Autodesk Inventor part; units mm, degrees
ref_plane "YZ Plane" through (0, 0, 0) normal (1, 0, 0) x (0, 1, 0)
ref_plane "XZ Plane" through (0, 0, 0) normal (0, 1, 0) x (-1, 0, 0)
ref_plane "XY Plane" through (0, 0, 0) normal (0, 0, 1) x (1, 0, 0)
sketch "Эскиз1" plane through (0, 0, 0) normal (0, 1, 0) x (-1, 0, 0)
  line L0 (0, 0) -> (12, 0)
  line L1 (12, 0) -> (12, -28)
  line L2 (12, -28) -> (0, -28)
  line L3 (0, -28) -> (0, 0)
  circle A0 centre (6, -12) radius 0.65
  circle A1 centre (6, -17) radius 2.5
  circle A2 centre (6, -22) radius 0.65
  line L4 (6, -12) -> (6, -17) construction
  line L5 (6, -17) -> (6, -22) construction
  line L6 (6, -6) -> (6, 0) construction
  line L7 (6, -12) -> (12, -12) construction
  circle A3 centre (6, -12) radius 1.15
  circle A4 centre (6, -22) radius 1.15
  line L8 (6, -22) -> (6, -28) construction
  line L9 (6, -12) -> (6, -6) construction
  point P0 (12, -14)
  dimension "d0" = 5
  dimension "d1" = 6
  dimension "d2" = 5
  dimension "d7" = 0.5
  dimension "d8" = 1.3
  dimension "d20" = 6
extrude "Выдавливание1" add sketch "Эскиз1" against normal blind 9 contours L0 L1 L2 L3 | A0 | A1 | A2 | A3 | A4
shell "Оболочка1" thickness 0.7 removed faces 1 at (-4, -9, -9.3333)
extrude "Выдавливание2" cut sketch "Эскиз1" against normal through all contours A0 | A1 | A2
sketch "Эскиз2" plane through (0, -9, 0) normal (0, -1, 0) x (1, 0, 0)
  line L0 (0, -28) -> (-12, -28) construction
  line L1 (-6, -28) -> (-6, 0) construction
  line L2 (-12, 0) -> (0, 0) construction
  line L3 (-12, -28) -> (-12, 0) construction
  line L4 (-12, -14) -> (0, -14) construction
  line L5 (0, 0) -> (0, -28) construction
  circle A0 centre (-1.1, -26.9) radius 0.9
  circle A1 centre (-1.1, -26.9) radius 0.5
  circle A2 centre (-10.9, -26.9) radius 0.9
  circle A3 centre (-10.9, -26.9) radius 0.5
  circle A4 centre (-1.1, -1.1) radius 0.9
  circle A5 centre (-1.1, -1.1) radius 0.5
  circle A6 centre (-10.9, -1.1) radius 0.5
  circle A7 centre (-10.9, -1.1) radius 0.9
  dimension "d11" = 1.1
  dimension "d12" = 1.1
  dimension "d13" = 1
  dimension "d14" = 0.4
extrude "Выдавливание3" cut sketch "Эскиз2" against normal through all contours A0 | A1 | A2 | A3 | A4 | A5 | A6 | A7
extrude "Выдавливание4" add sketch "Эскиз2" along normal blind 8.8 from surface at -9
fillet "Сопряжение1" radius 1 4 edges at (-12, -4.5, -28) (0, -4.5, -28) (0, -4.5, 0) (-12, -4.5, 0)
equation "\"d11\" = d12"
properties part number "Голова сервы"
Can you work these out from the model? Positions are in its coordinate system, mm. A direction names the side the tool comes from. Coordinates: 2 decimals unless noted, no trailing zeros. Loops run counter-clockwise (first coordinate to the right, second up) from the corner with the lowest first, then second, coordinate; pieces in that order, holes last.
1) Which directions (+Z, -Z, +X, -X, +Y, -Y) give clear straight access to the entire face, cutting with the end or side of a thin tool? Please do faces 1 (the flat face through (-6, -0.7, -14)), 2 (the cylindrical face through (-0.285, -4.563, -0.301)).
2) Imagine slicing it at D-D on x = -4.75. List the corners of the cut face in (y, z) for me, plus the area to 3 significant figures.
3) Thinking about a two-plate mould opening in Z: for faces 3 (the flat face through (-6, -4, -28)), 4 (the flat face through (-0.7, -5, -14)), 5 (the flat face through (-12, -4, -14)), which applies, pulls with the +Z half, pulls with the -Z half, needs draft (parallel to the pull), parting line crosses it, or undercut?
4) Imagine slicing it at A-A on y = -8. List the corners of the cut face in (x, z) for me.
5) I need wall thicknesses on probe 1 along Z at (x, y) = (-10.9, -4); probe 2 along Z at (x, y) = (-6, -0.2); probe 3 along X at (y, z) = (-5.5, -23.5). Which ranges of each line are inside material? Lowest first, please.
6) Imagine slicing it at B-B on x = -6. List the corners of the cut face in (y, z) for me, plus the area to 3 significant figures.
7) Imagine slicing it at C-C on z = -19. List the corners of the cut face in (x, y) for me, plus the area to 3 significant figures.
8) For pin 1 (3 mm diameter, centred on x = -3.5, z = -24, fed in from +Y); pin 2 (1.7 mm diameter, centred on x = -6, z = -22, fed in from -Y); pin 3 (1.1 mm diameter, centred on x = -10.9, z = -1.1, fed in from -Y); pin 4 (0.5 mm diameter, centred on x = -11, z = -27, fed in from -Y), each with a flat end and sliding along its axis, tell me the tip position at first contact or that it passes through.
Completed:
1. face 1: -Y
1. face 2: +Z, +X, +Y, -Y
2. outline: (-9, -28) - (0, -28) - (0, -19.17) - (-0.7, -19.17) - (-0.7, -27.3) - (-9, -27.3) - close; (-9, -0.7) - (-0.7, -0.7) - (-0.7, -14.83) - (0, -14.83) - (0, 0) - (-9, 0) - close
2. area: 28.2 mm2
3. face 3: pulls with the -Z half
3. face 4: undercut
3. face 5: needs draft
4. outline: (-12, -27) arc R1 ccw to (-11, -28) - (-1, -28) arc R1 ccw to (0, -27) - (0, -1) arc R1 ccw to (-1, 0) - (-11, 0) arc R1 ccw to (-12, -1) - close; hole circle Ø1 at (-10.9, -26.9); hole circle Ø1 at (-10.9, -1.1); hole (-11.3, -26.09) arc R0.9 cw to (-10.09, -27.3) - (-1.91, -27.3) arc R0.9 cw to (-0.7, -26.09) - (-0.7, -1.91) arc R0.9 cw to (-1.91, -0.7) - (-10.09, -0.7) arc R0.9 cw to (-11.3, -1.91) - close; hole circle Ø1 at (-1.1, -26.9); hole circle Ø1 at (-1.1, -1.1)
5. probe 1: z = -28 to -27.4, -26.4 to -26, -2 to -1.6, -0.6 to 0
5. probe 2: z = -28 to -22.65, -21.35 to -19.5, -14.5 to -12.65, -11.35 to 0
5. probe 3: x = -12 to -11.3, -0.7 to 0
6. outline: (-9, -28) - (0, -28) - (0, -22.65) - (-0.7, -22.65) - (-0.7, -27.3) - (-9, -27.3) - close; (-9, -0.7) - (-0.7, -0.7) - (-0.7, -11.35) - (0, -11.35) - (0, 0) - (-9, 0) - close; (-0.7, -21.35) - (0, -21.35) - (0, -19.5) - (-0.7, -19.5) - close; (-0.7, -14.5) - (0, -14.5) - (0, -12.65) - (-0.7, -12.65) - close
6. area: 25.9 mm2
7. outline: (-12, -9) - (-11.3, -9) - (-11.3, -0.7) - (-7.5, -0.7) - (-7.5, 0) - (-12, 0) - close; (-4.5, -0.7) - (-0.7, -0.7) - (-0.7, -9) - (0, -9) - (0, 0) - (-4.5, 0) - close
7. area: 17.9 mm2
8. pin 1: stops at y = 0
8. pin 2: stops at y = -0.7
8. pin 3: stops at y = -8.8
8. pin 4: passes through
